Autodesk Inventor part; units mm, degrees
ref_plane "YZ Plane" through (0, 0, 0) normal (1, 0, 0) x (0, 1, 0)
ref_plane "XZ Plane" through (0, 0, 0) normal (0, 1, 0) x (-1, 0, 0)
ref_plane "XY Plane" through (0, 0, 0) normal (0, 0, 1) x (1, 0, 0)
sketch "Sketch1" plane through (0, 0, 0) normal (0, 1, 0) x (-1, 0, 0)
  circle A0 centre (0, 0) radius 13.2908
  line L0 (0, 0) -> (-6.6454, 11.5102)
  line L1 (0, 0) -> (13.2908, 0) construction
  line L2 (0, 0) -> (-6.6454, -11.5102)
extrude "Extrusion1" add sketch "Sketch1" against normal blind 2.54
sketch "Sketch2" plane through (0, 0, 0) normal (0, 1, 0) x (1, 0, 0)
  line L0 (-12.5731, -2.5944) -> (-8.1825, -2.5944)
  line L1 (-8.1825, -2.5944) -> (-8.1825, 2.4614)
  line L2 (-8.1825, 2.4614) -> (-12.5731, 2.4614)
  line L3 (-12.5731, 2.4614) -> (-12.5731, -2.5944)
  line L4 (4.1689, -6.5202) -> (7.5172, -9.2912)
  line L5 (7.5172, -9.2912) -> (10.6841, -5.4645)
  line L6 (10.6841, -5.4645) -> (7.3357, -2.6935)
  line L7 (7.3357, -2.6935) -> (4.1689, -6.5202)
  line L8 (5.5175, 10.8555) -> (3.3095, 7.0709)
  line L9 (3.3095, 7.0709) -> (7.5616, 4.5902)
  line L10 (7.5616, 4.5902) -> (9.7696, 8.3747)
  line L11 (9.7696, 8.3747) -> (5.5175, 10.8555)
  point P0 (0, 0)
extrude "Extrusion2" add sketch "Sketch2" along normal blind 5.08
sketch "Sketch3" plane through (7.3357, 0, 2.6935) normal (0.6376, 0, -0.7704) x (-0.7704, 0, -0.6376)
  circle A0 centre (-2.0466, 2.54) radius 0.4266
  point P0 (7.3687, 0)
extrude "Extrusion3" add sketch "Sketch3" along normal blind 5.08
sketch "Sketch4" plane through (3.3095, 0, -7.0709) normal (-0.8637, 0, -0.5039) x (-0.5039, 0, 0.8637)
  circle A0 centre (-2.246, 2.54) radius 0.2524
  point P0 (7.7752, 0)
extrude "Extrusion4" add sketch "Sketch4" along normal blind 5.08
sketch "Sketch5" plane through (-12.5731, 0, 2.5944) normal (0, 0, 1) x (1, 0, 0)
  circle A0 centre (2.148, 2.6) radius 0.2719
  point P0 (12.5731, 0)
extrude "Extrusion5" add sketch "Sketch5" along normal blind 5.08
sketch "Sketch6" plane through (0, 0, 0) normal (0, 1, 0) x (1, 0, 0)
  point P0 (0, 0)
properties part number "Base"
Design review of the part built by this model. Coordinates are the model's own, in mm. A direction names the side the tool comes from. Round coordinates to 2 decimals unless told otherwise and drop trailing zeros. Write each loop counter-clockwise with the first axis right and the second up, starting at its lowest first coordinate (ties: lowest second). Pieces come first, ordered by that corner, then holes. Notation, with made-up numbers: (65, 48.5) -> (104, 48.5) arc R7 ccw to (104, 59.5) -> close; hole circle Ø9 at (80.25, -17). An arc over 180 degrees is marked (long way). One line per question, with ' | ' between items.
(1) Wall thickness on line 1 (X direction, y = 2.5, z = -10.75); line 2 (Y direction, x = -1.25, z = -5); line 3 (Z direction, x = 5.5, y = 4): over which ranges is each line inside the solid? List them lowest first. Write a range as [from, to].
Result sheet:
line 1: [0.97, 1.95], [5.46, 5.7] | line 2: [-2.54, 0] | line 3: [-10.83, -5.79], [4.91, 7.62]
(2) Take a section at D-D, the plane x = -0.5. State the section outline as (y, z) points, and give its area (3 significant figures).
Result sheet:
outline: (-2.54, -13.28) -> (0, -13.28) -> (0, 13.28) -> (-2.54, 13.28) -> close | area: 67.5 mm2
(3) Draft analysis for pull direction Y (two halves, no side actions). For faces 1 (the cylindrical face through (10.58, 2.956, 2.128)), 2 (the flat face through (7, 5.08, 6)), 3 (the flat face through (9.08, 2.5, 7.4)), state which applies: released by +Y, released by -Y, zero draft, split by the parting line, or undercut.
Result sheet:
face 1: undercut | face 2: released by +Y | face 3: zero draft
(4) Machinability: for faces 4 (the flat face through (5.406, 2.504, -5.848)), 5 (the flat face through (7.67, 2.5, -9.6)), 6 (the flat face through (-12.573, 3, 0)), 7 (the flat face through (-10, 3, -2.461)), 8 (the flat face through (8.65, 2.504, -6.456)), which of the approach directions +Z, -Z, +X, -X, +Y, -Y give a long, thin tool a straight path to every point of the face, cutting with its end or side? Answer none if there is none.
Result sheet:
face 4: -X, +Y | face 5: -Z, +X, +Y | face 6: +Z, -Z, -X, +Y | face 7: -Z, +X, -X, +Y | face 8: +X, +Y
(5) Insertion check: P1, Ø3, axis at y = 1, z = 2, coming from the -X side; P2, Ø1.3, axis at x = -10, y = 3.5, coming from the -Z side; P3, Ø2, axis at x = -10.5, y = 3.5, coming from the +Z side. Each pin has a flat end and moves straight along its axis. Give the tip position at first contact, or say it passes through.
Result sheet:
P1: x = -13.26 | P2: z = -2.46 | P3: z = 7.67
(6) Take a section at A-A, the plane y = 4.25. State the section outline as (x, z) points.
Result sheet:
outline: (-12.57, -2.46) -> (-8.18, -2.46) -> (-8.18, 2.59) -> (-12.57, 2.59) -> close; (3.31, -7.07) -> (5.52, -10.86) -> (9.77, -8.37) -> (7.56, -4.59) -> close; (4.17, 6.52) -> (7.34, 2.69) -> (10.68, 5.46) -> (7.52, 9.29) -> close
(7) Take a section at B-B, the plane x = 6.5. State the section outline as (y, z) points.
Result sheet:
outline: (-2.54, -11.59) -> (0, -11.59) -> (0, -10.28) -> (5.08, -10.28) -> (5.08, -5.21) -> (0, -5.21) -> (0, 3.7) -> (5.08, 3.7) -> (5.08, 8.45) -> (0, 8.45) -> (0, 11.59) -> (-2.54, 11.59) -> close
(8) Take a section at C-C, the plane y = -1. State the section outline as (x, z) points, and give its area (3 significant figures).
Result sheet:
outline: circle Ø26.58 at (0, 0) | area: 555 mm2
